Input: dimensioned drawing with shaded views. Units: mm. Origin: part minimum x, y, z. A direction names the side the tool comes from. Round coordinates to 2 decimals unless told otherwise and drop trailing zeros. Write each loop counter-clockwise with the first axis right and the second up, starting at its lowest first coordinate (ties: lowest second). Pieces come first, ordered by that corner, then holes. Notation, with made-up numbers: M 89.25,42 L 115.25,42 A30 ccw 115.25,70 Z; hole C -23.5,-11.75 d5. An arc over 180 degrees is marked long. Answer in a Markdown table with one row per item. Add a question column.
Item 1: Contact query for a flat-ended pin moving along its axis: pin 1 (3 mm diameter, centred on x = 27.5, y = 2, fed in from +Z). Output: stop coordinate, or through.
Item 2: Cut plane B-B on x = 24.5. Return loops of the section in (y, z).
Item 3: Material intervals for probe 1 along X at (y, z) = (1.35, 59) (1 decimal); probe 2 along Z at (x, y) = (30.5, 1.3); probe 3 along X at (y, z) = (1.7, 69), sorted ascending.
Item 4: Set-up query: the marked faces 1 and 2. Return all of +Z, -Z, +X, -X, +Y, -Y with unobstructed straight access to the full face (end or side cutting, diameter ignored); none if empty.
Item 5: Cut plane A-A on y = 3.9. Return loops of the section in (x, z).
Item 6: Mould query, pull axis X, two halves, no side actions, for the marked faces 3 and 4. Classes: released by +X, released by -X, zero draft, split by the parting line, or undercut.
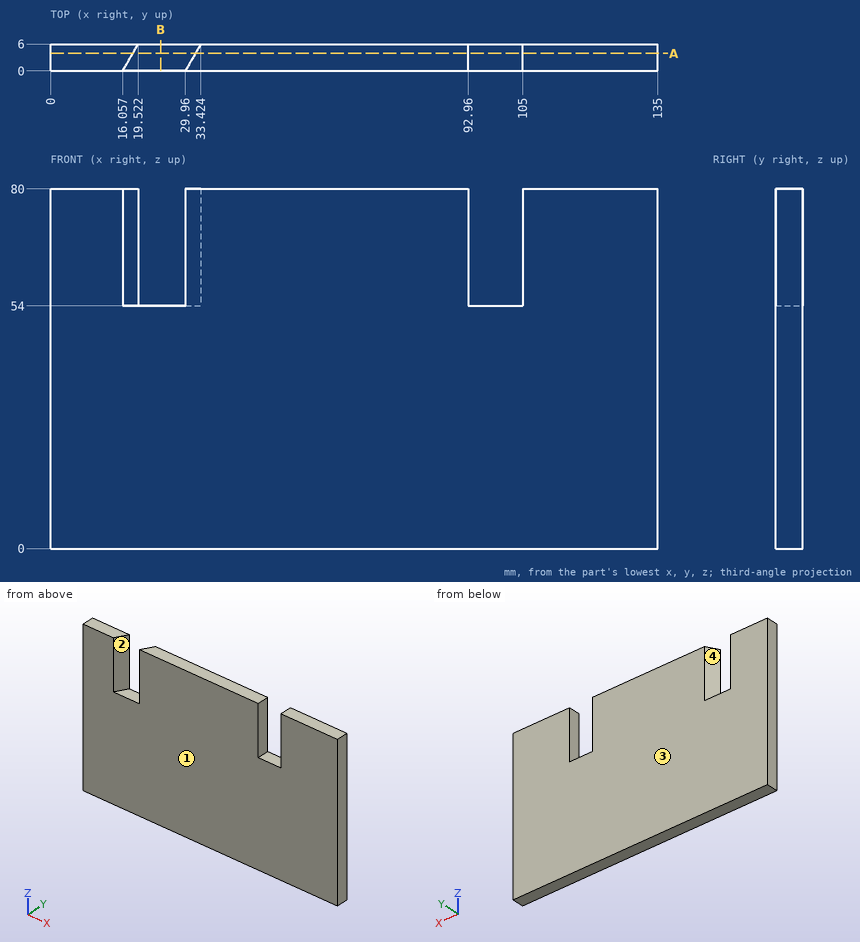
Results below:
| question | item | result |
|---|---|---|
| 1 | pin 1 | z = 54 |
| 2 | outline | M 0,0 L 6,0 L 6,54 L 0,54 Z |
| 3 | probe 1 | 0 to 16.8, 30.7 to 93, 105 to 135 |
| 3 | probe 2 | 0 to 54 |
| 3 | probe 3 | 0 to 17.04, 30.94 to 92.96, 105 to 135 |
| 4 | face 1 | +Z, -Z, +X, -X, -Y |
| 4 | face 2 | +Z, -Y |
| 5 | outline | M 0,0 L 135,0 L 135,80 L 105,80 L 105,54 L 92.96,54 L 92.96,80 L 32.21,80 L 32.21,54 L 18.31,54 L 18.31,80 L 0,80 Z |
| 6 | face 3 | zero draft |
| 6 | face 4 | undercut |
